Answer from the drawing. Dimensions are ordinates in mm from the lowest x, y and z of the part. Round coordinates to 2 decimals unless told otherwise and drop trailing zeros. Loops run counter-clockwise (first coordinate to the right, second up) from the corner with the lowest first, then second, coordinate; pieces in that order, holes last.
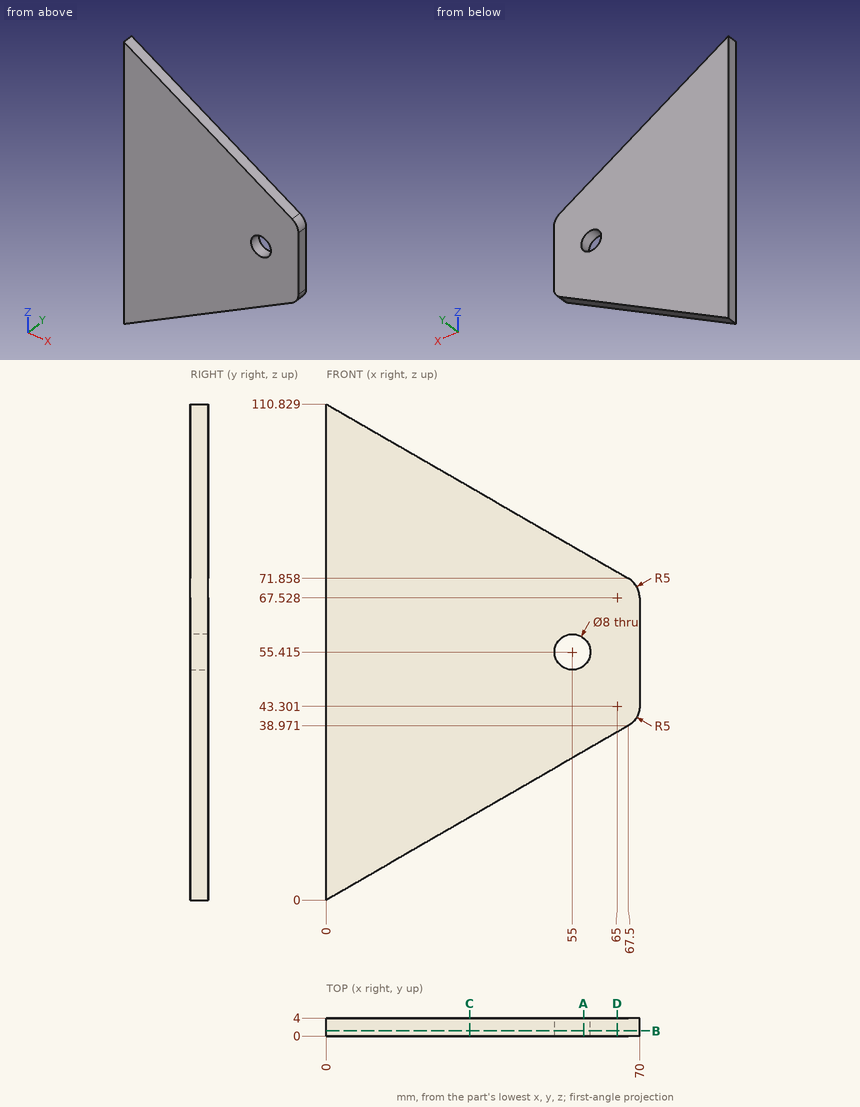
1. Find section B-B (y = 1.15). Write down the section's boundary in (x, z) (1 decimal), then the cut area to 3 significant figures.
Answer key:
outline: (0, 0) - (67.5, 39) arc R5 ccw to (70, 43.3) - (70, 67.5) arc R5 ccw to (67.5, 71.9) - (0, 110.8) - close; hole circle Ø8 at (55, 55.4)
area: 4,880 mm2
2. Given pin 1 (2 mm diameter, centred on y = 3, z = 52.5, fed in from -X); pin 2 (1 mm diameter, centred on y = 3, z = 96, fed in from +X); pin 3 (2 mm diameter, centred on x = 31.5, y = 2, fed in from -Z), each flat-ended and moving along its own axis, determine where each tip first touches the part or whether it passes through.
Answer key:
pin 1: stops at x = 0
pin 2: stops at x = 26.55
pin 3: stops at z = 17.61
3. Find section D-D (x = 65). Write down the section's boundary in (y, z).
Answer key:
outline: (0, 37.53) - (4, 37.53) - (4, 73.3) - (0, 73.3) - close
4. Find section C-C (x = 32). Write down the section's boundary in (y, z) (1 decimal).
Answer key:
outline: (0, 18.5) - (4, 18.5) - (4, 92.4) - (0, 92.4) - close
5. Consider probe 1 along Z at (x, y) = (53.5, 2.65) (1 decimal); probe 2 along Z at (x, y) = (52, 2.65) (1 decimal); probe 3 along X at (y, z) = (0.55, 22) (1 decimal). Determine where each line is inside the solid, lowest interval first.
Answer key:
probe 1: z = 30.9 to 51.7, 59.1 to 79.9
probe 2: z = 30 to 52.8, 58.1 to 80.8
probe 3: x = 0 to 38.1
6. Find section A-A (x = 57.5). Write down the section's boundary in (y, z), then the cut area to 3 significant figures.
Answer key:
outline: (0, 33.2) - (4, 33.2) - (4, 52.29) - (0, 52.29) - close; (0, 58.54) - (4, 58.54) - (4, 77.63) - (0, 77.63) - close
area: 153 mm2
